Build history of the part. All positions in model axes, mm. A direction names the side the tool comes from. Round coordinates to 2 decimals unless told otherwise and drop trailing zeros. Loops run counter-clockwise (first coordinate to the right, second up) from the corner with the lowest first, then second, coordinate; pieces in that order, holes last. Notation, with made-up numbers: (66.25, -36.5) -> (75.25, -36.5) arc R23 cw to (75.25, -12.5) -> close; hole circle Ø5 at (66, 33.5). An arc over 180 degrees is marked (long way). Put each result on its own line as item: value. Start each with the question number.
Item 1: Flat gauge pins, fed straight in: pin 1 Ø3 at (x, y) = (4, 13) entering from -Z; pin 2 Ø1.5 at (x, z) = (-0.5, -5.5) entering from -Y; pin 3 Ø1.8 at (y, z) = (19, 1) entering from +X; pin 4 Ø5 at (x, y) = (-1, 19) entering from -Z. Where does each tip first touch, or does it go through?
Item 2: Drill centre lines: probe 1 along X at (y, z) = (16.25, 0.5); probe 2 along X at (y, z) = (14.5, 0.5); probe 3 along Z at (x, y) = (-0.5, 25.75). Where is each one in solid material? Low to high. Write a range as [from, to].
Item 3: Pull direction Z, two halves, no side cores. Call faces 1 (the flat face through (0, 13, 7.243)), 2 (the cylindrical face through (0, 13.7, 2.6)), 3 (the flat face through (-7.243, 10, 0)): +Z half, -Z half, draft (parallel to the pull), parting line (faces both ways), or undercut.
Item 4: Cut at A-A, the plane y = 9.5. List the corners of the cut face in (x, z).
Item 5: Tool access for faces 4 (the flat face through (-1.55, 14, 0)), 5 (the flat face through (2, 0, 0)): list every direction of +Z, -Z, +X, -X, +Y, -Y with a clear straight run to the whole face (end or side of a thin tool).
Autodesk Inventor part; units mm, degrees
ref_plane "YZ Plane" through (0, 0, 0) normal (1, 0, 0) x (0, 1, 0)
ref_plane "XZ Plane" through (0, 0, 0) normal (0, 1, 0) x (-1, 0, 0)
ref_plane "XY Plane" through (0, 0, 0) normal (0, 0, 1) x (1, 0, 0)
sketch "Sketch3" plane through (0, 0, 0) normal (0, 1, 0) x (-1, 0, 0)
  line L0 (-3, -7.2426) -> (-7.2426, -3)
  line L1 (-7.2426, -3) -> (-7.2426, 3)
  line L2 (-7.2426, 3) -> (-3, 7.2426)
  line L3 (-3, 7.2426) -> (3, 7.2426)
  line L4 (3, 7.2426) -> (7.2426, 3)
  line L5 (7.2426, 3) -> (7.2426, -3)
  line L6 (7.2426, -3) -> (3, -7.2426)
  line L7 (3, -7.2426) -> (-3, -7.2426)
  point P0 (0, 0)
  point P1 (0, 0)
  dimension "d3" = 6
extrude "Extrusion2" add sketch "Sketch3" along normal blind 27
sketch "Sketch4" plane through (7.2426, 0, 3) normal (0.7071068, 0, 0.7071068) x (0.7071068, 0, -0.7071068)
  circle A0 centre (-3, 4.5) radius 2
  point P0 (-3, 0)
  dimension "d6" = 4
  dimension "d7" = 4.5
sketch "Sketch5" plane through (7.2426, 0, 3) normal (1, 0, 0) x (0, 0, -1)
  circle A0 centre (3, 13.5) radius 2
  point P0 (3, 0)
  dimension "d8" = 4
  dimension "d9" = 13.5
sketch "Sketch6" plane through (3, 0, -7.2426) normal (0.7071068, 0, -0.7071068) x (-0.7071068, 0, -0.7071068)
  circle A0 centre (-3, 4.5) radius 2
  circle A1 centre (-3, 13.5) radius 2
  point P0 (-3, 0)
  dimension "d10" = 4
  dimension "d11" = 4
  dimension "d12" = 4.5
  dimension "d13" = 9
sketch "Sketch7" plane through (3, 0, -7.2426) normal (0, 0, -1) x (-1, 0, 0)
  circle A0 centre (3, 22.5) radius 2
  point P0 (3, 0)
  dimension "d14" = 4
  dimension "d15" = 22.5
sketch "Sketch8" plane through (-7.2426, 0, -3) normal (-0.7071068, 0, -0.7071068) x (-0.7071068, 0, 0.7071068)
  circle A0 centre (-3, 4.5) radius 2
  circle A1 centre (-3, 22.5) radius 2
  point P0 (-3, 0)
  dimension "d16" = 4
  dimension "d17" = 4.5
  dimension "d18" = 4
  dimension "d19" = 22.5
sketch "Sketch9" plane through (-7.2426, 0, -3) normal (-1, 0, 0) x (0, 0, 1)
  circle A0 centre (3, 13.5) radius 2
  circle A1 centre (3, 22.5) radius 2
  point P0 (3, 0)
  dimension "d20" = 4
  dimension "d21" = 4
  dimension "d22" = 13.5
  dimension "d23" = 22.5
sketch "Sketch10" plane through (-3, 0, 7.2426) normal (-0.7071068, 0, 0.7071068) x (0.7071068, 0, 0.7071068)
  circle A0 centre (-3, 4.5) radius 2
  circle A1 centre (-3, 13.5) radius 2
  circle A2 centre (-3, 22.5) radius 2
  point P0 (-3, 0)
  dimension "d24" = 4
  dimension "d25" = 4
  dimension "d26" = 4
  dimension "d27" = 4.5
  dimension "d28" = 9
  dimension "d29" = 9
extrude "Extrusion3" add sketch "Sketch4" along normal blind 1
extrude "Extrusion4" add sketch "Sketch5" along normal blind 1
extrude "Extrusion5" add sketch "Sketch6" along normal blind 1
extrude "Extrusion6" add sketch "Sketch7" along normal blind 1
extrude "Extrusion7" add sketch "Sketch8" along normal blind 1
extrude "Extrusion8" add sketch "Sketch9" along normal blind 1
extrude "Extrusion9" add sketch "Sketch10" along normal blind 1
fillet "Fillet1" radius 2 12 edges at (-7.2426, 22.5, 4.4142) (-7.2426, 13.5, 4.4142) (-7.2426, 4.5, 4.4142) (-8.2426, 13.5, -2) (-8.2426, 22.5, -2) (-4.4142, 22.5, -7.2426) (-4.4142, 4.5, -7.2426) (2, 22.5, -8.2426) (7.2426, 13.5, -4.4142) (7.2426, 4.5, -4.4142) (8.2426, 13.5, 2) (4.4142, 4.5, 7.2426)
ref_plane "Work Plane1" through (7.2426, 27, -3) normal (0, 1, 0) x (0, 0, -1)
sketch "Sketch12" plane through (7.2426, 27, -3) normal (0, 1, 0) x (0, 0, -1)
  point P0 (-3, 7.2426)
sketch "Sketch13" plane through (7.2426, 27, -3) normal (0, 1, 0) x (0, 0, -1)
  circle A0 centre (-3, 7.2426) radius 2.6
  line L0 (-5.0875, 5.6926) -> (-0.9125, 5.6926)
  line L1 (-5.0875, 8.7926) -> (-0.9125, 8.7926)
  dimension "d52" = 5.2
  dimension "d53" = 1.55
  dimension "d54" = 1.55
extrude "Extrusion10" cut sketch "Sketch13" against normal blind 58.75 contours A0 L0 L1
properties part number "8-Lados"
Reply:
1. pin 1: stops at z = -7.24
1. pin 2: stops at y = 0
1. pin 3: stops at x = 7.24
1. pin 4: stops at z = -8.04
2. probe 1: x = [-7.24, -1.55], [1.55, 7.24]
2. probe 2: x = [-8.05, -1.55], [1.55, 8.05]
2. probe 3: z = [-7.24, -2.55], [2.55, 7.24]
3. face 1: +Z half
3. face 2: undercut
3. face 3: draft
4. outline: (-7.24, -3) -> (-3, -7.24) -> (3, -7.24) -> (7.24, -3) -> (7.24, 3) -> (3, 7.24) -> (-3, 7.24) -> (-7.24, 3) -> close; hole (-1.55, -2.09) arc R2.6 ccw to (1.55, -2.09) -> (1.55, 2.09) arc R2.6 ccw to (-1.55, 2.09) -> close
5. face 4: +Y, -Y
5. face 5: +Z, -Z, +X, -X, -Y
